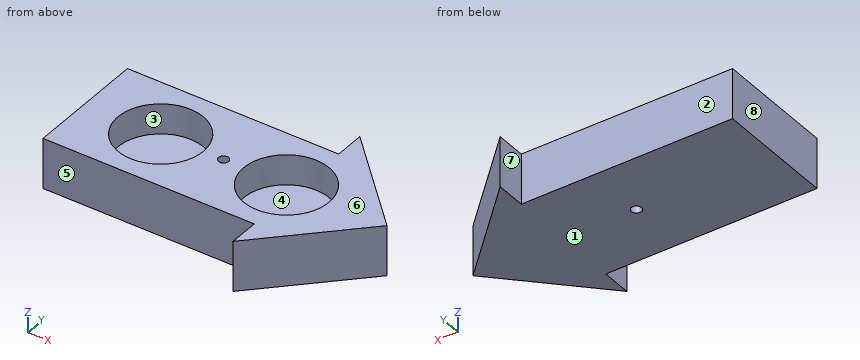
```python
from build123d import *

# Parameters (mm, degrees)
F0_W     = 42
F0_H     = 24
F1_DEPTH = 10
F2_R     = 8.5
F3_DEPTH = 6
F4_R     = 1
F5_DEPTH = 25


with BuildPart() as f1:
    # F0 (on Top) → F1 (new body)
    with BuildSketch(Plane.XY):
        with Locations((21, 12)):
            Rectangle(F0_W, F0_H)
        Polygon((42, 24), (42, 0), (42, -6), (60, 12), (42, 30), align=None)
    extrude(amount=F1_DEPTH)

    # F2 (on face) → F3 (cut)
    with BuildSketch(Plane.XY.offset(10)):
        with Locations((15, 12)):
            Circle(F2_R)
        with Locations((40, 12)):
            Circle(F2_R)
    extrude(amount=-F3_DEPTH, mode=Mode.SUBTRACT)

    # F4 (on face) → F5 (cut)
    with BuildSketch(Plane.XY.offset(10)):
        with Locations((27.5, 12)):
            Circle(F4_R)
    extrude(amount=-F5_DEPTH, mode=Mode.SUBTRACT)


solid = f1.part
```
CAD build for the part. Positions are in the model's coordinates, mm. Face numbers are marked on the shaded views. A direction names the side the tool comes from. Round coordinates to 2 decimals unless told otherwise and drop trailing zeros. Write each loop counter-clockwise with the first axis right and the second up, starting at its lowest first coordinate (ties: lowest second). Pieces come first, ordered by that corner, then holes.
Item 1: Drill centre lines: L1, parallel to Y at x = 27.5, z = 6; L2, parallel to Y at x = 40, z = 7.25; L3, parallel to Z at x = 12, y = 11.5. Where is each one in solid material? Low to high.
Filled in:
L1: y = 0 to 11, 13 to 24
L2: y = 0 to 3.5, 20.5 to 24
L3: z = 0 to 4
Item 2: Band-saw the part on B-B on z = 9. Write the cut outline in (x, y), then the cut area to 3 significant figures.
Filled in:
outline: (0, 0) - (42, 0) - (42, -6) - (60, 12) - (42, 30) - (42, 24) - (0, 24) - close; hole circle Ø17 at (15, 12); hole circle Ø2 at (27.5, 12); hole circle Ø17 at (40, 12)
area: 875 mm2
Item 3: Band-saw the part on C-C on x = 15. Write the cut outline in (y, z).
Filled in:
outline: (0, 0) - (24, 0) - (24, 10) - (20.5, 10) - (20.5, 4) - (3.5, 4) - (3.5, 10) - (0, 10) - close
Item 4: Tool access for the marked faces 4, 5, 6, 7 and 8: list every direction of +Z, -Z, +X, -X, +Y, -Y with a clear straight run to the whole face (end or side of a thin tool).
Filled in:
face 4: +Z
face 5: +Z, -Z, -X, -Y
face 6: +Z, +X, -X, +Y, -Y
face 7: +Z, -Z, -X, +Y
face 8: +Z, -Z, -X, +Y, -Y
Item 5: Mould opens along Y. For the marked faces 1, 2 and 3 say: released by +Y, released by -Y, zero draft, split by the parting line, or undercut.
Filled in:
face 1: zero draft
face 2: released by +Y
face 3: undercut
Item 6: Drop flat-ended pins along their axis: pin 1 Ø1 at (x, z) = (28, 4) entering from +Y; pin 2 Ø1.8 at (y, z) = (-2, 2.5) entering from -X; pin 3 Ø3 at (x, z) = (47, 8.5) entering from +Y. Give the stop position or say it passes through.
Filled in:
pin 1: stops at y = 24
pin 2: stops at x = 42
pin 3: stops at y = 26.5
Item 7: Band-saw the part on A-A on x = 27.5. Write the cut outline in (y, z).
Filled in:
outline: (0, 0) - (11, 0) - (11, 10) - (0, 10) - close; (13, 0) - (24, 0) - (24, 10) - (13, 10) - close
Item 8: Band-saw the part on D-D on y = 1. Write the cut outline in (x, z).
Filled in:
outline: (0, 0) - (49, 0) - (49, 10) - (0, 10) - close
